The drawing under review shows one solid part. Ordinate dimensions are in mm from its lowest x, y, z. A direction names the side the tool comes from. Round coordinates to 2 decimals unless told otherwise and drop trailing zeros. Write each loop counter-clockwise with the first axis right and the second up, starting at its lowest first coordinate (ties: lowest second). Pieces come first, ordered by that corner, then holes. Notation, with made-up numbers: M 20.5,26.25 L 56.5,26.25 A27 cw 56.5,43.25 Z; hole C -15,-26.75 d4. An arc over 180 degrees is marked long. One line per item, written item: value. Start each with the question number.
1) Take a section at D-D, the plane z = 19.25. Write out the cut boundary in (x, y).
2) Wall thickness on probe 1 along Z at (x, y) = (47, 22); probe 2 along X at (y, z) = (6.5, 4); probe 3 along X at (y, z) = (8.5, 5): over which ranges is each line inside the solid? List them lowest first.
3) Take a section at A-A, the plane y = 41.5. Write out the cut boundary in (x, z), and give its area (3 significant figures).
4) Tool access review of the marked faces 1, 2 and 3: name each direction out of +Z, -Z, +X, -X, +Y, -Y from which nothing blocks a thin tool from reaching the whole face with its end or side.
5) Take a section at C-C, the plane x = 25. Write out the cut boundary in (y, z), and give its area (3 significant figures).
6) For P1, Ø4, axis at x = 17.5, z = 13.5, coming from the +Y side; P2, Ø20, axis at x = 29, y = 35, coming from the +Z side; P3, Ø5, axis at x = 26.5, z = 7, coming from the +Y side, all flat-tipped, find the tip position at first contact; note any pin that passes through.
7) Take a section at B-B, the plane z = 5.75. Write out the cut boundary in (x, y).
8) Mouldability with a two-part tool opening along X and no side actions: class the marked faces 4, 5 and 6 as +X half, -X half, draft (parallel to the pull), parting line (faces both ways), or undercut.
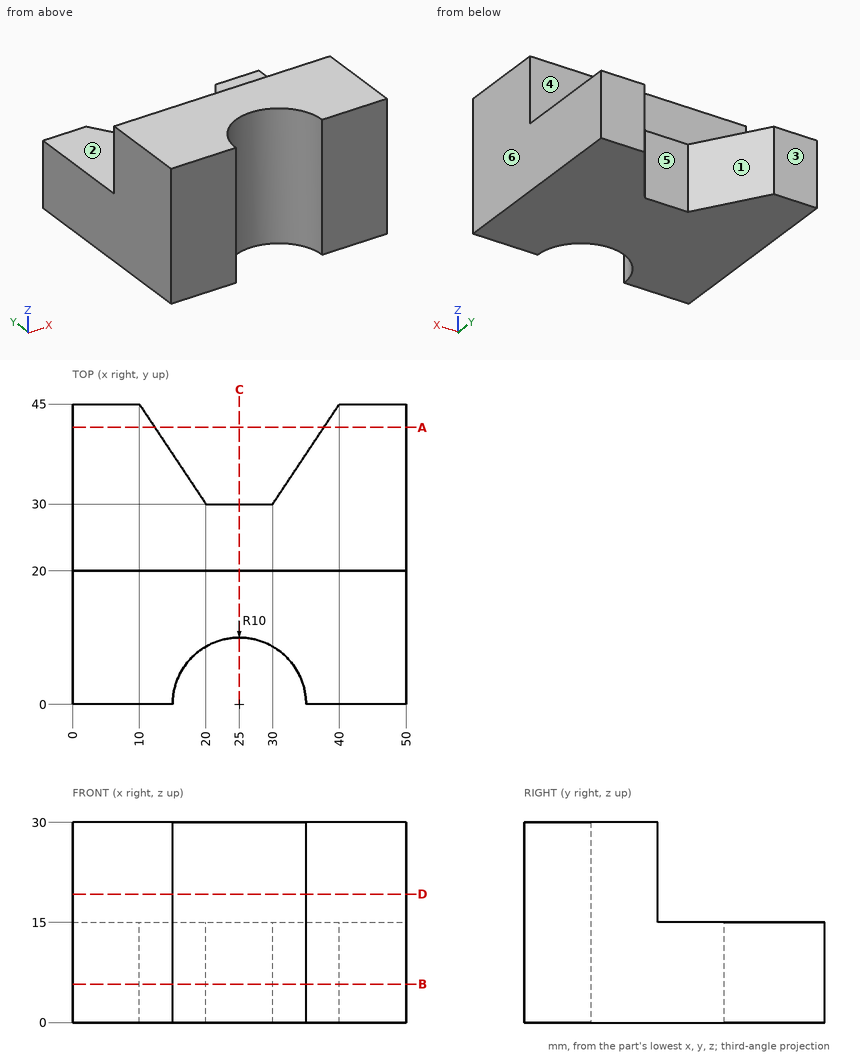
Checked values:
1. outline: M 0,0 L 15,0 A10 cw 35,0 L 50,0 L 50,20 L 0,20 Z
2. probe 1: z = 0 to 15
2. probe 2: x = 0 to 17.4, 32.6 to 50
2. probe 3: x = 0 to 19.73, 30.27 to 50
3. outline: M 0,0 L 12.33,0 L 12.33,15 L 0,15 Z; M 37.67,0 L 50,0 L 50,15 L 37.67,15 Z
3. area: 370 mm2
4. face 1: +Z, -Z, +Y
4. face 2: +Z, +X, -X, +Y
4. face 3: +Z, -Z, +X, -X, +Y
5. outline: M 10,0 L 30,0 L 30,15 L 20,15 L 20,30 L 10,30 Z
5. area: 450 mm2
6. P1: stops at y = 36.75
6. P2: stops at z = 15
6. P3: stops at y = 30
7. outline: M 0,0 L 15,0 A10 cw 35,0 L 50,0 L 50,45 L 40,45 L 30,30 L 20,30 L 10,45 L 0,45 Z
8. face 4: draft
8. face 5: undercut
8. face 6: +X half
